Part model, mm, in its own coordinate system. Face numbers are marked on the shaded views. A direction names the side the tool comes from. Give positions to 0.01 mm unless a question says otherwise; leave off trailing zeros. Order: outer loops, then holes, each group sorted by start corner. A loop starts at its lowest first (then second) coordinate and runs counter-clockwise, first axis right, second up. Notation, with made-up numbers: (-33.5, 62.25) - (-21.5, 62.25) arc R24 cw to (-21.5, 98.25) - close; hole circle Ø10 at (32, -40). An arc over 180 degrees is marked (long way). Use a Markdown table: item, result. Add a question column.
from build123d import *


with BuildPart() as part:
    # Sketch1 → Revolve1 (revolve)
    with BuildSketch(Plane(origin=(0, 0, 0), x_dir=(0, 0, -1), z_dir=(1, 0, 0)), mode=Mode.PRIVATE) as revolve1_sk:
        with BuildLine():
            Line((-33.715360463, 3.5), (-28.715360463, 3.5))
            Line((-28.715360463, 3.5), (10.584639537, 11.1))
            Line((10.584639537, 11.1), (17.084639537, 11.1))
            Line((17.084639537, 11.1), (17.084639537, 25))
            Line((17.084639537, 25), (12.084639537, 25))
            ThreePointArc((12.084639537, 25), (9.735819432, 18.5466698), (3.788398149, 15.112924521))
            Line((3.788398149, 15.112924521), (-33.715360463, 8.5))
            Line((-33.715360463, 8.5), (-33.715360463, 3.5))
        make_face()
    revolve(revolve1_sk.sketch.rotate(Axis((0, 0, 51.495497957), (0, 0, -1)), 90), axis=Axis((0, 0, 51.495497957), (0, 0, -1)))


solid = part.part
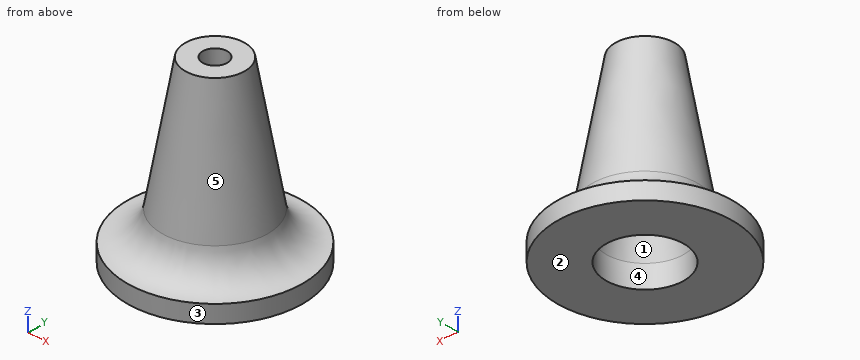
1. Cut at A-A (y = 0). Write the cut outline in (x, z), plus the area to 3 significant figures.
2. Cut at D-D (z = 4). Write the cut outline in (x, y).
3. Mould opens along X. For the marked faces 1, 2 and 3 say: released by +X, released by -X, zero draft, split by the parting line, or undercut.
4. Pin check, flat tips, straight feed: P1, Ø6, axis at x = 6, z = 16, coming from the -Y side; P2, Ø5, axis at y = 4, z = 4.5, coming from the -X side; P3, Ø10, axis at y = -2.5, z = 6, coming from the +X side. Stop position of each tip, or through.
5. Tool access for the marked faces 4 and 5: list every direction of +Z, -Z, +X, -X, +Y, -Y with a clear straight run to the whole face (end or side of a thin tool).
6. Drill centre lines: probe 1 along Y at (x, z) = (0, -15); probe 2 along Y at (x, z) = (0, 31.25); probe 3 along X at (y, z) = (-4, -8). Where is each one in solid material? Low to high. Write a range as [from, to].
7. Cut at C-C (z = -13). Write the cut outline in (x, y).
Responses:
| question | item | result |
|---|---|---|
| 1 | outline | (-25, -17.08) - (-11.1, -17.08) - (-11.1, -10.58) - (-3.5, 28.72) - (-3.5, 33.72) - (-8.5, 33.72) - (-15.11, -3.79) arc R10.04 cw to (-25, -12.08) - close; (3.5, 28.72) - (11.1, -10.58) - (11.1, -17.08) - (25, -17.08) - (25, -12.08) arc R10.04 cw to (15.11, -3.79) - (8.5, 33.72) - (3.5, 33.72) - close |
| 1 | area | 674 mm² |
| 2 | outline | circle Ø27.48 at (0, 0); hole circle Ø16.56 at (0, 0) |
| 3 | face 1 | undercut |
| 3 | face 2 | zero draft |
| 3 | face 3 | split by the parting line |
| 4 | P1 | stops at y = -11.39 |
| 4 | P2 | stops at x = -13.78 |
| 4 | P3 | stops at x = 14.19 |
| 5 | face 4 | -Z |
| 5 | face 5 | +Z |
| 6 | probe 1 | y = [-25, -11.1], [11.1, 25] |
| 6 | probe 2 | y = [-8.93, -3.5], [3.5, 8.93] |
| 6 | probe 3 | x = [-16.44, -9.82], [9.82, 16.44] |
| 7 | outline | circle Ø50 at (0, 0); hole circle Ø22.2 at (0, 0) |
